```python
from build123d import *

# Parameters (mm, degrees)
F1_W     = 240
F1_H     = 240
F1_W_2   = 6
F1_H_2   = 6
F1_W_3   = 208
F1_H_3   = 208
F2_DEPTH = 3
F3_DEPTH = 25
F8_W     = 40
F8_H     = 15
F8_R     = 4
F9_DEPTH = 3


with BuildPart() as f2:
    # F1 (on Front) → F2 (new body)
    with BuildSketch(Plane.XZ):
        with Locations((120, 120)):
            Rectangle(F1_W, F1_H)
        with Locations((6, 234)):
            Rectangle(F1_W_2, F1_H_2, mode=Mode.SUBTRACT)
        with Locations((120, 120)):
            Rectangle(F1_W_3, F1_H_3, mode=Mode.SUBTRACT)
        with Locations((6, 234)):
            Rectangle(F1_W_2, F1_H_2)
    extrude(amount=F2_DEPTH)

    # F1 (on Front) → F3 (cut)
    with BuildSketch(Plane.XZ):
        with Locations((6, 234)):
            Rectangle(F1_W_2, F1_H_2)
    extrude(amount=F3_DEPTH, mode=Mode.SUBTRACT)

    # F5: F2 across plane


with BuildPart() as f2_1:
    add(f2.part)
    add(f2.part.mirror(Plane(origin=(120, -1.5, 120), x_dir=(0, -1, 0), z_dir=(-1, 0, 0))), mode=Mode.INTERSECT)

    # F7: F2 across plane


with BuildPart() as f2_2:
    add(f2_1.part)
    add(f2_1.part.mirror(Plane(origin=(120, -1.5, 120), x_dir=(1, 0, 0), z_dir=(0, 0, 1))), mode=Mode.INTERSECT)

    # F8 (on face) → F9 (join)
    with BuildSketch(Plane.XZ.offset(3)):
        with Locations((54, 23.5)):
            Rectangle(F8_W, F8_H)
        with Locations((44, 23.5)):
            Circle(F8_R, mode=Mode.SUBTRACT)
        with Locations((64, 23.5)):
            Circle(F8_R, mode=Mode.SUBTRACT)
    extrude(amount=-F9_DEPTH)


solid = f2_2.part
```
For this review, take the finished solid that the model builds, in its own axes (mm). Round coordinates to 2 decimals unless told otherwise and drop trailing zeros. Write each loop counter-clockwise with the first axis right and the second up, starting at its lowest first coordinate (ties: lowest second). Pieces come first, ordered by that corner, then holes. Notation, with made-up numbers: (29.5, -26.75) - (86.5, -26.75) arc R20 ccw to (86.5, -21.75) - close; hole circle Ø1 at (20, -5). An arc over 180 degrees is marked (long way). Put each result on its own line as item: value.
Q1. Mouldability with a two-part tool opening along X and no side actions: class faces 1 (the face through (67.815, -1.521, 24.701)), 2 (the face through (225, 0, 122)) as released by +X, released by -X, zero draft, split by the parting line, or undercut.
Solved:
face 1: undercut
face 2: zero draft
Q2. We need section A-A (x = 139.5). Give the boundary of the cut face in (y, z), and give its area (3 significant figures).
Solved:
outline: (-3, 0) - (0, 0) - (0, 16) - (-3, 16) - close; (-3, 224) - (0, 224) - (0, 240) - (-3, 240) - close
area: 96.0 mm2
Q3. We need section D-D (z = 202). Give the boundary of the cut face in (x, y).
Solved:
outline: (0, -3) - (16, -3) - (16, 0) - (0, 0) - close; (224, -3) - (240, -3) - (240, 0) - (224, 0) - close
Q4. Wall thickness on probe 1 along Z at (x, y) = (44, -1.7); probe 2 along X at (y, z) = (-2.05, 32.5); probe 3 along Z at (x, y) = (41, -0.65): over which ranges is each line inside the solid? List them lowest first.
Solved:
probe 1: z = 0 to 19.5, 27.5 to 31, 224 to 240
probe 2: x = 0 to 16, 224 to 240
probe 3: z = 0 to 20.85, 26.15 to 31, 224 to 240
Q5. We need section C-C (z = 23.5). Give the boundary of the cut face in (x, y).
Solved:
outline: (0, -3) - (16, -3) - (16, 0) - (0, 0) - close; (34, -3) - (40, -3) - (40, 0) - (34, 0) - close; (48, -3) - (60, -3) - (60, 0) - (48, 0) - close; (68, -3) - (74, -3) - (74, 0) - (68, 0) - close; (224, -3) - (240, -3) - (240, 0) - (224, 0) - close
Q6. We need section B-B (x = 64). Give the boundary of the cut face in (y, z).
Solved:
outline: (-3, 0) - (0, 0) - (0, 19.5) - (-3, 19.5) - close; (-3, 27.5) - (0, 27.5) - (0, 31) - (-3, 31) - close; (-3, 224) - (0, 224) - (0, 240) - (-3, 240) - close
